from build123d import *

# Parameters (mm, degrees)
SKETCH_1_R           = 2.25
EXTRUDE_1_DEPTH      = 38
SKETCH_2_W           = 1.5
SKETCH_2_H           = 38
EXTRUDE_2_DEPTH      = 8
EXTRUDE_2_DEPTH_BACK = 3
SKETCH_3_W           = 8
SKETCH_3_H           = 38
EXTRUDE_3_DEPTH      = 1.5


with BuildPart() as part:
    # 草圖1 → 填料-伸長1 (new body)
    with BuildSketch(Plane(origin=(0, 0, 0), x_dir=(1, 0, 0), z_dir=(0, 1, 0))):
        Circle(SKETCH_1_R)
    extrude(amount=EXTRUDE_1_DEPTH)

    # 草圖2 → 填料-伸長2 (add, two sides)
    with BuildSketch(Plane(origin=(3, 0, 0), x_dir=(0, 0, -1), z_dir=(1, 0, 0))) as extrude_2_sk:
        with Locations((0, 19)):
            Rectangle(SKETCH_2_W, SKETCH_2_H)
    extrude(amount=EXTRUDE_2_DEPTH)
    extrude(extrude_2_sk.sketch, amount=-EXTRUDE_2_DEPTH_BACK)

    # 草圖3 → 填料-伸長3 (add)
    with BuildSketch(Plane(origin=(11, 0, 0), x_dir=(0, 0, -1), z_dir=(1, 0, 0))):
        with Locations((0, 19)):
            Rectangle(SKETCH_3_W, SKETCH_3_H)
    extrude(amount=EXTRUDE_3_DEPTH)


solid = part.part
Design review of the part built by this model. Coordinates are the model's own, in mm. A direction names the side the tool comes from. Give positions to 0.01 mm unless a question says otherwise; leave off trailing zeros. Order: outer loops, then holes, each group sorted by start corner. A loop starts at its lowest first (then second) coordinate and runs counter-clockwise, first axis right, second up. Notation, with made-up numbers: (27.25, -28.5) - (47.25, -28.5) arc R25 cw to (47.25, 5.5) - close; hole circle Ø1 at (82, 36.25). An arc over 180 degrees is marked (long way). Write item = value, one per line. Start each with the question number.
Q1. We need section A-A on y = 12.5. State the section outline as (x, z) points.
Q2. Clearance check with flat-ended pins moving along their axes: pin 1 Ø1.5 at (x, y) = (8.5, 19.5) entering from -Z; pin 2 Ø7 at (x, y) = (4.5, 18) entering from -Z. State where each tip first meets the part, or that it passes through.
Q3. Tool access review of faces 1 (the face through (7, 19, -0.75)), 2 (the face through (6, 38, 0)), 3 (the face through (11, 19, 2)): name each direction out of +Z, -Z, +X, -X, +Y, -Y from which nothing blocks a thin tool from reaching the whole face with its end or side.
Q4. We need section C-C on z = 3. State the section outline as (x, y) points.
Q5. Mouldability with a two-part tool opening along X and no side actions: class faces 4 (the face through (12.5, 19, 0)), 5 (the face through (-2.25, 18.73, -0.09)), 6 (the face through (6, 0, 0)) as released by +X, released by -X, zero draft, split by the parting line, or undercut.
Q6. To check wall thickness, follow L1, parallel to Z at x = 6.5, y = 6.5; L2, parallel to X at y = 21, z = -3.5; L3, parallel to X at y = 14, z = -2. State the ranges of each line that lie inside material, in increasing order. Write a range as from..to.
Q7. We need section B-B on x = 0. State the section outline as (y, z) points.
Working result:
q1.outline = (2.12, -0.75) - (11, -0.75) - (11, -4) - (12.5, -4) - (12.5, 4) - (11, 4) - (11, 0.75) - (2.12, 0.75) arc R2.25 ccw (long way) to start
q2.pin_1 = -0.75
q2.pin_2 = -2.02
q3.face_1 = -Z, +Y, -Y
q3.face_2 = +Z, -Z, +X, -X, +Y
q3.face_3 = +Z, +Y, -Y
q4.outline = (11, 0) - (12.5, 0) - (12.5, 38) - (11, 38) - close
q5.face_4 = released by +X
q5.face_5 = undercut
q5.face_6 = zero draft
q6.L1 = -0.75..0.75
q6.L2 = 11..12.5
q6.L3 = -1.03..1.03, 11..12.5
q7.outline = (0, -2.25) - (38, -2.25) - (38, 2.25) - (0, 2.25) - close
